Part model, mm, in its own coordinate system. A direction names the side the tool comes from. Round coordinates to 2 decimals unless told otherwise and drop trailing zeros. Loops run counter-clockwise (first coordinate to the right, second up) from the corner with the lowest first, then second, coordinate; pieces in that order, holes last.
(1) Cut at D-D on x = 37. List the corners of the cut face in (y, z).
(2) Tool access for faces 4 (the face through (11, 30, -12.7)), 5 (the face through (11, 27.781, -6)), 6 (the face through (12.38, 3.15, -3.47)): list every direction of +Z, -Z, +X, -X, +Y, -Y with a clear straight run to the whole face (end or side of a thin tool).
(3) Cut at A-A on x = 6.5. List the corners of the cut face in (y, z), then the cut area to 3 significant figures.
(4) Probe probe 1 along Y at (x, z) = (-1.5, -57.15); probe 2 along Z at (x, y) = (25.5, 42); probe 3 along Z at (x, y) = (2, 15.5). List the from-to ranges inside material, lowest first.
(5) Cut at C-C on y = 18.5. List the corners of the cut face in (x, z), then the cut area to 3 significant figures.
(6) Flat gauge pins, fed straight in: pin 1 (1 mm diameter, centred on y = 8.5, z = -46, fed in from -X); pin 2 (4 mm diameter, centred on x = -2.5, y = 19, fed in from -Z); pin 3 (6.5 mm diameter, centred on x = 13.5, z = -10, fed in from +Y); pin 4 (5 mm diameter, centred on x = 13.5, y = 22, fed in from -Z). Where does each tip first touch, or does it go through?
(7) Mould opens along X. For faces 1 (the face through (14, 1.588, -10)), 2 (the face through (-7.938, 28.2, -57.2)), 3 (the face through (4, 14, 0)) say: +X half, -X half, draft (parallel to the pull), parting line (faces both ways), or undercut.
(8) Cut at B-B on z = -57.15. List the corners of the cut face in (x, y), then the cut area to 3 significant figures.
Autodesk Inventor part; units mm, degrees
ref_plane "YZ Plane" through (0, 0, 0) normal (1, 0, 0) x (0, 1, 0)
ref_plane "XZ Plane" through (0, 0, 0) normal (0, 1, 0) x (-1, 0, 0)
ref_plane "XY Plane" through (0, 0, 0) normal (0, 0, 1) x (1, 0, 0)
sketch "Sketch1" plane through (0, 0, 0) normal (1, 0, 0) x (0, 1, 0)
  line L0 (0, 0) -> (32.5438, 0)
  line L1 (32.5438, 0) -> (32.5438, -63.5)
  line L2 (32.5438, -63.5) -> (0, -63.5)
  line L3 (0, -63.5) -> (0, 0)
  dimension "d0" = 32.5438
  dimension "d1" = 63.5
extrude "Extrusion1" add sketch "Sketch1" along normal blind 4.7625
sketch "Sketch2" plane through (4.7625, 0, 0) normal (1, 0, 0) x (0, 0, -1)
  line L0 (0, 32.5438) -> (0, 0)
  line L1 (0, 0) -> (63.5, 0)
  line L2 (63.5, 0) -> (63.5, 32.5438)
  line L3 (63.5, 32.5438) -> (0, 32.5438)
  line L4 (0, 32.5438) -> (12.7, 32.5438)
  line L5 (12.7, 32.5438) -> (12.7, 27.7812)
  line L6 (12.7, 27.7812) -> (0, 27.7812)
  line L7 (0, 27.7812) -> (0, 32.5438)
  dimension "d4" = 12.7
  dimension "d5" = 4.7625
extrude "Extrusion2" add sketch "Sketch2" along normal blind 12.7 contours L3 L5 L6 L0
sketch "Sketch3" plane through (4.7625, 0, 0) normal (1, 0, 0) x (0, 0, -1)
  line L0 (12.7, 27.7812) -> (0, 27.7812)
  line L1 (0, 27.7812) -> (0, 0)
  line L2 (0, 0) -> (63.5, 0)
  line L3 (63.5, 0) -> (63.5, 32.5438)
  line L4 (63.5, 32.5438) -> (12.7, 32.5438)
  line L5 (12.7, 32.5438) -> (12.7, 27.7812)
  line L6 (0, 0) -> (25.4, 0)
  line L7 (25.4, 0) -> (25.4, 4.7625)
  line L8 (25.4, 4.7625) -> (0, 4.7625)
  line L9 (0, 4.7625) -> (0, 0)
  dimension "d8" = 4.7625
extrude "Extrusion3" add sketch "Sketch3" along normal blind 25.4 contours L8 L7 L2 L1
sketch "Sketch4" plane through (0, 0, 0) normal (-1, 0, 0) x (0, 0, 1)
  line L0 (0, 0) -> (0, 32.5438)
  line L1 (0, 32.5438) -> (-63.5, 32.5438)
  line L2 (-63.5, 32.5438) -> (-63.5, 0)
  line L3 (-63.5, 0) -> (0, 0)
  line L4 (-63.5, 32.5438) -> (-12.7, 32.5438)
  line L5 (-63.5, 32.5438) -> (-50.8, 32.5438)
  line L6 (-50.8, 32.5438) -> (-50.8, 16.6688)
  line L7 (-50.8, 16.6688) -> (-63.5, 16.6688)
  line L8 (-63.5, 16.6688) -> (-63.5, 32.5438)
  dimension "d11" = 12.7
  dimension "d12" = 15.875
extrude "Extrusion4" add sketch "Sketch4" along normal blind 7.9375 contours L2 L1 L6 L7
sketch "Sketch5" plane through (4.7625, 0, 0) normal (1, 0, 0) x (0, 0, -1)
  line L0 (25.4, 4.7625) -> (25.4, 0)
  line L1 (25.4, 0) -> (63.5, 0)
  line L2 (63.5, 0) -> (63.5, 32.5438)
  line L3 (63.5, 32.5438) -> (12.7, 32.5438)
  line L4 (12.7, 32.5438) -> (12.7, 27.7812)
  line L5 (12.7, 27.7812) -> (0, 27.7812)
  line L6 (0, 27.7812) -> (0, 4.7625)
  line L7 (0, 4.7625) -> (25.4, 4.7625)
  line L8 (0, 32.5438) -> (0, 27.7812)
  line L9 (0, 27.7812) -> (12.7, 27.7812)
  line L10 (12.7, 27.7812) -> (12.7, 32.5438)
  line L11 (12.7, 32.5438) -> (0, 32.5438)
  point P0 (0, 0)
  point P1 (57.15, 24.6063)
  dimension "d15" = 4.7625
  dimension "d16" = 7.9375
  dimension "d17" = 6.35
hole "Hole1" at (4.7625, 24.6063, -57.15) direction (-1, 0, 0) diameter 6.858 end through all
sketch "Sketch6" plane through (4.7625, 4.7625, 0) normal (0, 1, 0) x (1, 0, 0)
  line L0 (0, 0) -> (0, 25.4)
  line L1 (0, 0) -> (25.4, 0)
  line L2 (25.4, 25.4) -> (25.4, 0)
  line L3 (0, 25.4) -> (25.4, 25.4)
  point P0 (-4.7625, 0)
  point P1 (9.525, 9.525)
  dimension "d25" = 9.525
  dimension "d26" = 9.525
hole "Hole2" at (14.2875, 4.7625, -9.525) direction (0, -1, 0) diameter 12.7 depth 3.175
sketch "Sketch8" plane through (4.7625, 0, 0) normal (1, 0, 0) x (0, 0, -1)
  circle A0 centre (57.15, 24.6063) radius 3.429
  line L0 (25.4, 4.7625) -> (25.4, 0)
  line L1 (25.4, 0) -> (63.5, 0)
  line L2 (63.5, 0) -> (63.5, 32.5438)
  line L3 (63.5, 32.5438) -> (12.7, 32.5438)
  line L4 (12.7, 32.5438) -> (12.7, 27.7812)
  line L5 (12.7, 27.7812) -> (0, 27.7812)
  line L6 (0, 27.7812) -> (0, 4.7625)
  line L7 (0, 4.7625) -> (25.4, 4.7625)
  line L8 (63.5, 32.5438) -> (77.7875, 70.6438)
  line L9 (63.5, 32.5438) -> (104.1908, 32.5438) construction
  line L10 (77.7875, 70.6438) -> (82.55, 70.6438)
  line L11 (82.55, 70.6438) -> (82.55, 26.1938)
  line L12 (82.55, 26.1938) -> (77.7875, 26.1938)
  line L13 (77.7875, 26.1938) -> (77.7875, 70.6438)
  line L14 (77.7875, 26.1938) -> (63.5, 26.1938)
  point P0 (0, 0)
  dimension "d39" = 4.7625
  dimension "d40" = 44.45
  dimension "d41" = 38.1
  dimension "d47" = 25.4
extrude "Extrusion6" add sketch "Sketch8" against normal blind 4.7625 contours L2 L8 L13 L14 | L13 L10 L11 L12
sketch "Sketch9" plane through (4.7625, 0, 0) normal (1, 0, 0) x (0, 0, -1)
  circle A0 centre (57.15, 24.6063) radius 3.429
  line L0 (25.4, 4.7625) -> (25.4, 0)
  line L1 (25.4, 0) -> (63.5, 0)
  line L2 (63.5, 0) -> (63.5, 26.1938)
  line L3 (63.5, 26.1938) -> (82.55, 26.1938)
  line L4 (82.55, 26.1938) -> (82.55, 70.6438)
  line L5 (82.55, 70.6438) -> (77.7875, 70.6438)
  line L6 (77.7875, 70.6438) -> (63.5, 32.5438)
  line L7 (63.5, 32.5438) -> (12.7, 32.5438)
  line L8 (12.7, 32.5438) -> (12.7, 27.7812)
  line L9 (12.7, 27.7812) -> (0, 27.7812)
  line L10 (0, 27.7812) -> (0, 4.7625)
  line L11 (0, 4.7625) -> (25.4, 4.7625)
  line L12 (77.7875, 70.6438) -> (82.55, 70.6438)
  line L13 (82.55, 38.8938) -> (82.55, 70.6438)
  line L14 (82.55, 26.1938) -> (82.55, 70.6438)
  line L15 (77.7875, 70.6438) -> (82.55, 70.6438)
  line L16 (82.55, 70.6438) -> (82.55, 26.1938)
  line L17 (82.55, 26.1938) -> (77.7875, 26.1938)
  line L18 (77.7875, 26.1938) -> (77.7875, 70.6438)
  point P0 (0, 0)
  point P1 (88.9, 26.1938)
extrude "Extrusion7" add sketch "Sketch9" along normal blind 38.1 contours L18 L5 L4 L3
fillet "Fillet1" radius 6.35 1 edges at (2.3813, 26.1938, -63.5)
properties part number "WheelIntake4.0Base"
Final values:
1. outline: (26.19, -82.55) - (70.64, -82.55) - (70.64, -77.79) - (26.19, -77.79) - close
2. face 4: +X, +Y
2. face 5: +Z, +X
2. face 6: none
3. outline: (0, -25.4) - (4.76, -25.4) - (4.76, 0) - (0, 0) - close; (26.19, -82.55) - (70.64, -82.55) - (70.64, -77.79) - (26.19, -77.79) - close; (27.78, -12.7) - (32.54, -12.7) - (32.54, 0) - (27.78, 0) - close
3. area: 393 mm2
4. probe 1: y = 16.67 to 21.18, 28.04 to 32.54
4. probe 2: z = -82.55 to -77.79
4. probe 3: z = -63.5 to 0
5. outline: (-7.94, -63.5) - (4.76, -63.5) - (4.76, 0) - (0, 0) - (0, -50.8) - (-7.94, -50.8) - close
5. area: 403 mm2
6. pin 1: stops at x = 0
6. pin 2: stops at z = -63.5
6. pin 3: stops at y = 32.54
6. pin 4: passes through
7. face 1: undercut
7. face 2: -X half
7. face 3: draft
8. outline: (-7.94, 16.67) - (0, 16.67) - (0, 0) - (4.76, 0) - (4.76, 21.18) - (-7.94, 21.18) - close; (-7.94, 28.04) - (4.76, 28.04) - (4.76, 32.54) - (-7.94, 32.54) - close
8. area: 194 mm2
